from build123d import *

# Parameters (mm, degrees)
SKETCH1_R           = 44.45
SKETCH1_R_2         = 31.75
BOSS_EXTRUDE1_DEPTH = 50.8
SKETCH3_R           = 5.5
CUT_EXTRUDE2_DEPTH  = 8.5


with BuildPart() as part:
    # Sketch1 → Boss-Extrude1 (new body)
    with BuildSketch(Plane(origin=(0, 0, 0), x_dir=(1, 0, 0), z_dir=(0, 1, 0))):
        Circle(SKETCH1_R)
        Circle(SKETCH1_R_2, mode=Mode.SUBTRACT)
    extrude(amount=BOSS_EXTRUDE1_DEPTH)

    # Sketch3 → Cut-Extrude2 (cut)
    with BuildSketch(Plane(origin=(0, 50.8, 0), x_dir=(1, 0, 0), z_dir=(0, 1, 0))):
        with Locations((-28.145825623, 16.25)):
            Circle(SKETCH3_R)
        with Locations((0, -32.5)):
            Circle(SKETCH3_R)
        with Locations((28.145825623, 16.25)):
            Circle(SKETCH3_R)
    extrude(amount=-CUT_EXTRUDE2_DEPTH, mode=Mode.SUBTRACT)


solid = part.part
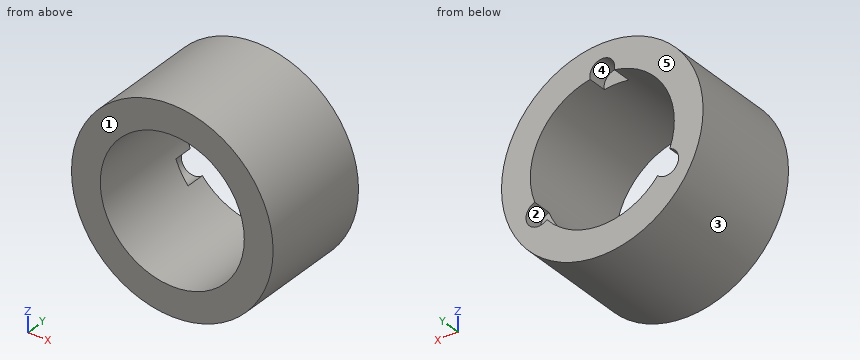
Part model, mm, in its own coordinate system. Face numbers are marked on the shaded views. A direction names the side the tool comes from. Coordinates: 2 decimals unless noted, no trailing zeros. Loops run counter-clockwise (first coordinate to the right, second up) from the corner with the lowest first, then second, coordinate; pieces in that order, holes last. Notation, with made-up numbers: M 19,-9 L 32,-9 A11 ccw 32,6 Z; hole C -2,12 d5. An arc over 180 degrees is marked long. Use a Markdown table: item, result. Add a question column.
Q1. Mould opens along X. For the marked faces 3, 4 and 5 say: +X half, -X half, draft (parallel to the pull), parting line (faces both ways), or undercut.
Q2. Probe L1, parallel to Z at x = 0, y = 48.5; L2, parallel to Z at x = -1, y = 8; L3, parallel to X at y = 35, z = 15. List the from-to ranges inside material, lowest first.
Q3. Pin check, flat tips, straight feed: P1, Ø10, axis at x = 12, y = 17, coming from the -Z side; P2, Ø5.5, axis at x = -0.5, z = 34.5, coming from the +Y side; P3, Ø12, axis at x = -19.5, z = -27, coming from the -Y side; P4, Ø5, axis at x = -33, y = 40.5, coming from the -Z side (3 decimals). Stop position of each tip, or through.
Q4. Cut at D-D (x = 11). Write the cut outline in (y, z), and give its area (3 significant figures).
Q5. Which spindle directions (+Z, -Z, +X, -X, +Y, -Y) get a long thin tool onto all of the face, cutting with end or side? Do the marked faces 1 and 2. Say none if no direction does.
Q6. Cut at B-B (x = 0). Write the cut outline in (y, z), and give its area (3 significant figures).
Q7. Cut at C-C (z = 36). Write the cut outline in (x, y).
Q8. Cut at A-A (z = 0). Write the cut outline in (x, y), and give its area (3 significant figures).
Worked out:
| question | item | result |
|---|---|---|
| 1 | face 3 | parting line |
| 1 | face 4 | undercut |
| 1 | face 5 | draft |
| 2 | L1 | z = -44.45 to -31.75, 38 to 44.45 |
| 2 | L2 | z = -44.44 to -31.73, 31.73 to 44.44 |
| 2 | L3 | x = -41.84 to -27.98, 27.98 to 41.84 |
| 3 | P1 | stops at z = -43.9 |
| 3 | P2 | stops at y = 42.3 |
| 3 | P3 | stops at y = 0 |
| 3 | P4 | stops at z = -32.335 |
| 4 | outline | M 0,-43.07 L 50.8,-43.07 L 50.8,-29.78 L 0,-29.78 Z; M 0,29.78 L 50.8,29.78 L 50.8,43.07 L 0,43.07 Z |
| 4 | area | 1,350 mm2 |
| 5 | face 1 | +Z, -Z, +X, -X, -Y |
| 5 | face 2 | +Y |
| 6 | outline | M 0,-44.45 L 50.8,-44.45 L 50.8,-31.75 L 0,-31.75 Z; M 0,31.75 L 42.3,31.75 L 42.3,38 L 50.8,38 L 50.8,44.45 L 0,44.45 Z |
| 6 | area | 1,240 mm2 |
| 7 | outline | M -26.07,0 L 26.07,0 L 26.07,50.8 L 4.24,50.8 L 4.24,42.3 L -4.24,42.3 L -4.24,50.8 L -26.07,50.8 Z |
| 8 | outline | M -44.45,0 L -31.75,0 L -31.75,50.8 L -44.45,50.8 Z; M 31.75,0 L 44.45,0 L 44.45,50.8 L 31.75,50.8 Z |
| 8 | area | 1,290 mm2 |
